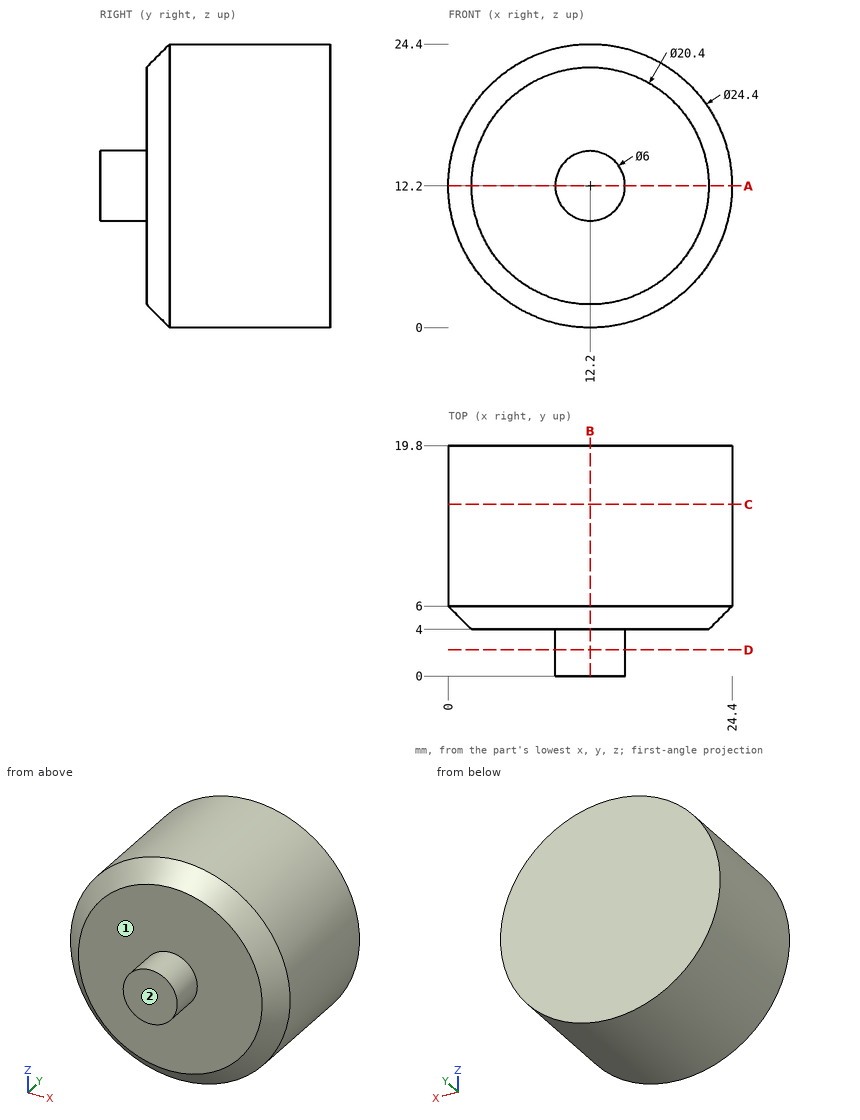
Print and shaded views of the part. All mm, measured from the part's lowest x, y and z. A direction names the side the tool comes from. Coordinates: 2 decimals unless noted, no trailing zeros. Write each loop counter-clockwise with the first axis right and the second up, starting at its lowest first coordinate (ties: lowest second). Pieces come first, ordered by that corner, then holes. Notation, with made-up numbers: (30, 88.25) - (89, 88.25) arc R35 cw to (89, 123.25) - close; hole circle Ø9 at (2, -27.5). An arc over 180 degrees is marked (long way). One line per question, with ' | ' between items. Start each with the question number.
Q1. Cut at B-B, the plane x = 12.2. List the corners of the cut face in (y, z).
Q2. Drill centre lines: line 1 (Y direction, x = 20.5, z = 14); line 2 (Z direction, x = 12, y = 18.5); line 3 (Z direction, x = 9.5, y = 11.25). Where is each one in solid material? Low to high. Write a range as [from, to].
Q3. Cut at C-C, the plane y = 14.75. List the corners of the cut face in (x, z), then the cut area to 3 significant figures.
Q4. Pin check, flat tips, straight feed: pin 1 (1 mm diameter, centred on y = 15, z = 9.5, fed in from -X); pin 2 (2 mm diameter, centred on y = 9.5, z = 10.5, fed in from +X); pin 3 (8 mm diameter, centred on y = 2.5, z = 18, fed in from +X). Stop position of each tip, or through.
Q5. 3-axis set-ups, long thin cutter, end or side, ignore diameter. For the marked faces 1 and 2: which of +Z, -Z, +X, -X, +Y, -Y reach the whole face in a straight line?
Q6. Cut at D-D, the plane y = 2.25. List the corners of the cut face in (x, z), then the cut area to 3 significant figures.
Q7. Cut at A-A, the plane z = 12.2. List the corners of the cut face in (x, y), then the cut area to 3 significant figures.
Answer below:
1) outline: (0, 9.2) - (4, 9.2) - (4, 2) - (6, 0) - (19.8, 0) - (19.8, 24.4) - (6, 24.4) - (4, 22.4) - (4, 15.2) - (0, 15.2) - close
2) line 1: [4, 19.8] | line 2: [0, 24.4] | line 3: [0.3, 24.1]
3) outline: circle Ø24.4 at (12.2, 12.2) | area: 468 mm^2
4) pin 1: x = 0.2 | pin 2: x = 24.38 | pin 3: x = 23.77
5) face 1: -Y | face 2: +Z, -Z, +X, -X, -Y
6) outline: circle Ø6 at (12.2, 12.2) | area: 28.3 mm^2
7) outline: (0, 6) - (2, 4) - (9.2, 4) - (9.2, 0) - (15.2, 0) - (15.2, 4) - (22.4, 4) - (24.4, 6) - (24.4, 19.8) - (0, 19.8) - close | area: 406 mm^2
